Part model, mm, in its own coordinate system. A direction names the side the tool comes from. Give positions to 0.01 mm unless a question says otherwise; leave off trailing zeros. Write each loop counter-clockwise with the first axis right and the second up, starting at its lowest first coordinate (ties: lowest second). Pieces come first, ordered by that corner, then holes.
Autodesk Inventor part; units mm, degrees
ref_plane "Work Plane1" through (0, 0, 0) normal (-1, 0, 0) x (0, 0, 1)
ref_plane "YZ Plane" through (0, 0, 0) normal (1, 0, 0) x (0, 1, 0)
ref_plane "XZ Plane" through (0, 0, 0) normal (0, 1, 0) x (-1, 0, 0)
sketch "Sketch1" plane through (0, 0, 0) normal (1, 0, 0) x (0, 1, 0)
  line L0 (67.821, 0) -> (56.1452, -2.7707)
  line L1 (67.821, 0) -> (0, 0)
  dimension "d2" = 12
  dimension "d10" = 67.821
ref_plane "Work Plane1" through (0, 0, 0) normal (-1, 0, 0) x (0, 0, 1)
sketch "Sketch2" plane through (0, 0, 0) normal (-1, 0, 0) x (0, 0, 1)
  line L0 (0, 67.821) -> (0, 83.821)
  line L1 (-13.5147, 54.1452) -> (-13.5147, 49.7452)
  arc A0 (-11.5147, 56.1452) -> (-13.5147, 54.1452) centre (-11.5147, 54.1452) ccw
  line L2 (0, 67.821) -> (0, 58.1452)
  arc A1 (-2, 56.1452) -> (0, 58.1452) centre (-2, 58.1452) ccw
  line L3 (-2, 56.1452) -> (-11.5147, 56.1452)
  point P0 (-13.5147, 56.1452)
  dimension "d5" = 16
  dimension "d12" = 6.4
  dimension "d13" = 2
  dimension "d16" = 2
ref_plane "Work Plane2" through (0, 83.821, 0) normal (0, 1, 0) x (-1, 0, 0)
sketch "Sketch3" plane through (0, 83.821, 0) normal (0, 1, 0) x (-1, 0, 0)
  circle A0 centre (0, 0) radius 0.45
  dimension "d6" = 0.9
sweep "Sweep3" add profiles "Sketch3" path "Sketch2"
properties part number "cable 2"
1) Saw through at A-A, the plane x = -0.05. Write the cut outline in (y, z).
Answers follow:
outline: (49.75, -13.96) - (54.15, -13.96) arc R2.45 ccw to (56.59, -11.51) - (56.59, -2) arc R1.55 cw to (58.15, -0.45) - (83.82, -0.45) - (83.82, 0.45) - (58.15, 0.45) arc R2.45 ccw to (55.7, -2) - (55.7, -11.51) arc R1.55 cw to (54.15, -13.07) - (49.75, -13.07) - close
2) Saw through at C-C, the plane z = -8.75. Write the cut outline in (x, y), then the cut area to 3 significant figures.
Answers follow:
outline: circle Ø0.9 at (0, 56.15)
area: 0.636 mm2
3) Wall check: L1, parallel to Z at x = 0.05, y = 81; L2, parallel to Y at x = 0.05, z = -11.25; L3, parallel to Y at x = 0.4, z = -6.75. Give the ranges that are in metal, low to high.
Answers follow:
L1: z = -0.45 to 0.45
L2: y = 55.7 to 56.59
L3: y = 55.94 to 56.35
4) Saw through at B-B, the plane y = 66.5. Write the cut outline in (x, z).
Answers follow:
outline: circle Ø0.9 at (0, 0)
5) Pin check, flat tip, straight feed: pin 1 Ø8 at (y, z) = (59.5, -11.5) entering from +X. Stop position of the tip, or through.
Answers follow:
pin 1: stops at x = 0.45
6) 3-axis set-ups, long thin cutter, end or side, ignore diameter. For faces 1 (the face through (-0.242, 55.766, -6.691)), 2 (the face through (0.098, 51.976, -13.954)), 3 (the face through (0, 49.745, -13.5)), 4 (the face through (-0.429, 71.163, 0.135)), 5 (the face through (0, 83.821, 0)): which of +Z, -Z, +X, -X, +Y, -Y reach the whole face in a straight line?
Answers follow:
face 1: none
face 2: -Y
face 3: +Z, -Z, +X, -X, -Y
face 4: +Y
face 5: +Z, -Z, +X, -X, +Y
